Source: CAD feature listing. Evaluate the final solid. Frame: model axes, mm. A direction names the side the tool comes from. Give positions to 0.01 mm unless a question says otherwise; leave off trailing zeros. Order: outer loops, then holes, each group sorted by start corner. A loop starts at its lowest first (then second) coordinate and runs counter-clockwise, first axis right, second up. Notation, with made-up numbers: M 14.25,87.25 L 30.25,87.25 A23 ccw 30.25,102.25 Z; hole C 35.5,33.25 d4. An arc over 180 degrees is marked long. Use CSV: the item, a comma, the result in double quotes. Start each with the question number.
1. Section query B-B, the plane z = 8.75. Return the cut outline in (x, y), plus the area to 3 significant figures.
2. Section query A-A, the plane y = 47.55. Return the cut outline in (x, z).
3. Reachability of faces 5 (the flat face through (-52, 11, 0)), 6 (the flat face through (47, -13.65, -4)), 7 (the flat face through (52, -37, 0)), 8 (the flat face through (-45, 3.45, -4)) from +Z, -Z, +X, -X, +Y, -Y: full face, straight path, thin tool, end or side. Return the list, or none.
4. Pin query (flat end, axial travel): P1, Ø7, axis at y = 22.5, z = -5.5, coming from the -X side; P2, Ø2, axis at x = -35, z = -3, coming from the -Y side; P3, Ø15, axis at x = 48.5, z = -5, coming from the -Y side; P4, Ø8.5, axis at y = 39, z = -6.5, coming from the +X side. Return the tip coordinate at first contact, or that it passes through.
5. Line query: line 1 along Y through (x, z) = (45.35, 0.7); line 2 along Y through (x, z) = (49.5, -5); line 3 along X through (y, z) = (3.5, 9.75). Output: solid intervals per line, ascending. Write a range as [from, to].
6. Section query C-C, the plane x = 13. Return the cut outline in (y, z), plus the area to 3 significant figures.
7. Section query D-D, the plane y = 30.5. Return the cut outline in (x, z), plus the area to 3 significant figures.
8. Mould query, pull axis Y, two halves, no side actions, for faces 1 (the flat face through (-37.15, -11, -4)), 2 (the flat face through (-51, -28.45, -4)), 3 (the flat face through (-49, -31.85, -3)), 4 (the flat face through (-49, 43.15, -4)). Classes: released by +Y, released by -Y, zero draft, split by the parting line, or undercut.
from build123d import *

# Parameters (mm, degrees)
SKETCH_1_W          = 101.7
SKETCH_1_H          = 101.7
EXTRUDE_1_DEPTH     = 1.5
SKETCH_2_R          = 1.5
CUT_EXTRUDE_1_DEPTH = 2.5
SKETCH_3_W          = 11.5
SKETCH_3_H          = 7.6
SKETCH_3_W_2        = 9
SKETCH_3_H_2        = 9.3
SKETCH_3_W_3        = 16.7
SKETCH_3_H_3        = 14.8
SKETCH_3_W_4        = 5.5
SKETCH_3_H_4        = 6
SKETCH_3_W_5        = 14
SKETCH_3_H_5        = 9.1
SKETCH_3_W_6        = 11.7
SKETCH_3_H_6        = 10
SKETCH_3_W_7        = 15
SKETCH_3_H_7        = 16.2
SKETCH_3_W_8        = 12.5
SKETCH_3_H_8        = 15
SKETCH_3_H_9        = 7.35
EXTRUDE_2_DEPTH     = 9
SKETCH_4_W          = 9
SKETCH_4_H          = 9.3
CUT_EXTRUDE_2_DEPTH = 4.1
SKETCH_5_W          = 16.7
SKETCH_5_H          = 14.8
CUT_EXTRUDE_3_DEPTH = 0.3
SKETCH_7_W          = 14
SKETCH_7_H          = 9.1
CUT_EXTRUDE_4_DEPTH = 3
SKETCH_8_W          = 15
SKETCH_8_H          = 16.2
EXTRUDE_4_DEPTH     = 13.5
SKETCH_9_W          = 89
SKETCH_9_H          = 53.5
EXTRUDE_5_DEPTH     = 17
FILLET_1_R          = 10


with BuildPart() as part:
    # 草图1 → 凸台-拉伸1 (new body)
    with BuildSketch(Plane.XY):
        Rectangle(SKETCH_1_W, SKETCH_1_H)
    extrude(amount=EXTRUDE_1_DEPTH)

    # 草图2 → 切除-拉伸1 (cut, through all)
    with BuildSketch(Plane(origin=(0, 0, 0), x_dir=(-1, 0, 0), z_dir=(0, 0, -1))):
        with Locations((-45.35, -47.55)):
            Circle(SKETCH_2_R)
        with Locations((45.35, -47.55)):
            Circle(SKETCH_2_R)
        with Locations((45.35, 47.55)):
            Circle(SKETCH_2_R)
        with Locations((-45.35, 47.55)):
            Circle(SKETCH_2_R)
    extrude(amount=-CUT_EXTRUDE_1_DEPTH, mode=Mode.SUBTRACT)

    # 草图3 → 凸台-拉伸2 (add)
    with BuildSketch(Plane(origin=(0, 0, 0), x_dir=(-1, 0, 0), z_dir=(0, 0, -1))):
        with Locations((49.1, 39.35)):
            Rectangle(SKETCH_3_W, SKETCH_3_H)
        with Locations((49.05, 28.95)):
            Rectangle(SKETCH_3_W_2, SKETCH_3_H_2)
        with Locations((45.5, 10.85)):
            Rectangle(SKETCH_3_W_3, SKETCH_3_H_3)
        with Locations((45.5, -11.28)):
            Rectangle(SKETCH_3_W_3, SKETCH_3_H_3)
        with Locations((51.3, -25.45)):
            Rectangle(SKETCH_3_W_4, SKETCH_3_H_4)
        with Locations((48.95, -36.4)):
            Rectangle(SKETCH_3_W_5, SKETCH_3_H_5)
        with Locations((-46.2, 38.26)):
            Rectangle(SKETCH_3_W_6, SKETCH_3_H_6)
        with Locations((-46.15, 20.19)):
            Rectangle(SKETCH_3_W_7, SKETCH_3_H_7)
        with Locations((-46.15, 0.32)):
            Rectangle(SKETCH_3_W_7, SKETCH_3_H_7)
        with Locations((-47.4, -21.15)):
            Rectangle(SKETCH_3_W_8, SKETCH_3_H_8)
        with Locations((-47.8, -37.545)):
            Rectangle(SKETCH_3_W_6, SKETCH_3_H_9)
    extrude(amount=EXTRUDE_2_DEPTH)

    # 草图4 → 切除-拉伸2 (cut)
    with BuildSketch(Plane(origin=(0, 0, -9), x_dir=(-1, 0, 0), z_dir=(0, 0, -1))):
        with Locations((49.05, 28.95)):
            Rectangle(SKETCH_4_W, SKETCH_4_H)
    extrude(amount=-CUT_EXTRUDE_2_DEPTH, mode=Mode.SUBTRACT)

    # 草图5 → 切除-拉伸3 (cut)
    with BuildSketch(Plane(origin=(0, 0, -9), x_dir=(-1, 0, 0), z_dir=(0, 0, -1))):
        with Locations((45.5, 10.85)):
            Rectangle(SKETCH_5_W, SKETCH_5_H)
        with Locations((45.5, -11.28)):
            Rectangle(SKETCH_5_W, SKETCH_5_H)
    extrude(amount=-CUT_EXTRUDE_3_DEPTH, mode=Mode.SUBTRACT)

    # 草图7 → 切除-拉伸4 (cut)
    with BuildSketch(Plane(origin=(0, 0, -9), x_dir=(-1, 0, 0), z_dir=(0, 0, -1))):
        with Locations((48.95, -36.4)):
            Rectangle(SKETCH_7_W, SKETCH_7_H)
    extrude(amount=-CUT_EXTRUDE_4_DEPTH, mode=Mode.SUBTRACT)

    # 草图8 → 凸台-拉伸4 (add)
    with BuildSketch(Plane(origin=(0, 0, -9), x_dir=(-1, 0, 0), z_dir=(0, 0, -1))):
        with Locations((-46.15, 0.32)):
            Rectangle(SKETCH_8_W, SKETCH_8_H)
        with Locations((-46.15, 20.19)):
            Rectangle(SKETCH_8_W, SKETCH_8_H)
    extrude(amount=-EXTRUDE_4_DEPTH)

    # 草图9 → 凸台-拉伸5 (add)
    with BuildSketch(Plane.XY.offset(1.5)):
        with Locations((6.15, -10.8)):
            Rectangle(SKETCH_9_W, SKETCH_9_H)
    extrude(amount=EXTRUDE_5_DEPTH)

    # 圆角1
    fillet_1_edges = [part.edges().sort_by_distance(p)[0] for p in [
        (-38.35, 15.95, 10),
        (-38.35, -37.55, 10),
    ]]
    fillet(fillet_1_edges, radius=FILLET_1_R)


solid = part.part
Result set:
1,outline,"M -38.35,-27.55 A10 ccw -28.35,-37.55 L 50.65,-37.55 L 50.65,15.95 L -28.35,15.95 A10 ccw -38.35,5.95 Z"
1,area,"4,720 mm2"
2,outline,"M -50.85,0 L -46.85,0 L -46.85,1.5 L -50.85,1.5 Z; M -43.85,0 L 43.85,0 L 43.85,1.5 L -43.85,1.5 Z; M 46.85,0 L 50.85,0 L 50.85,1.5 L 46.85,1.5 Z"
3,face 5,"+Z, -X, +Y, -Y"
3,face 6,"-Z, +X"
3,face 7,"+Z, +X, -Y"
3,face 8,"-Z, -X"
4,P1,"x = -53.55"
4,P2,"through"
4,P3,"y = -50.85"
4,P4,"x = 52.05"
5,line 1,"[-50.85, -49.05], [-46.05, 46.05], [49.05, 50.85]"
5,line 2,"[-41.22, -33.87], [-28.65, -13.65], [-7.78, 8.42], [12.09, 28.29], [33.26, 43.26]"
5,line 3,"[-38.35, 50.65]"
6,outline,"M -50.85,0 L 50.85,0 L 50.85,1.5 L 15.95,1.5 L 15.95,18.5 L -37.55,18.5 L -37.55,1.5 L -50.85,1.5 Z"
6,area,"1,060 mm2"
7,outline,"M -53.55,-4.9 L -44.55,-4.9 L -44.55,0 L 50.85,0 L 50.85,1.5 L -50.85,1.5 L -50.85,0 L -53.55,0 Z"
7,area,"197 mm2"
8,face 1,"zero draft"
8,face 2,"undercut"
8,face 3,"undercut"
8,face 4,"released by +Y"
